Input: dimensioned drawing with shaded views. Units: mm. Origin: part minimum x, y, z. Give positions to 0.01 mm unless a question says otherwise; leave off trailing zeros. Write each loop counter-clockwise with the first axis right and the second up, starting at its lowest first coordinate (ties: lowest second). Pieces come first, ordered by that corner, then holes. Notation, with made-up numbers: (7.5, 6) -> (23.5, 6) arc R28 cw to (23.5, 29) -> close; hole circle Ø4 at (75, -8). An arc over 180 degrees is marked (long way). Answer as a JSON object with one key per item and string values.
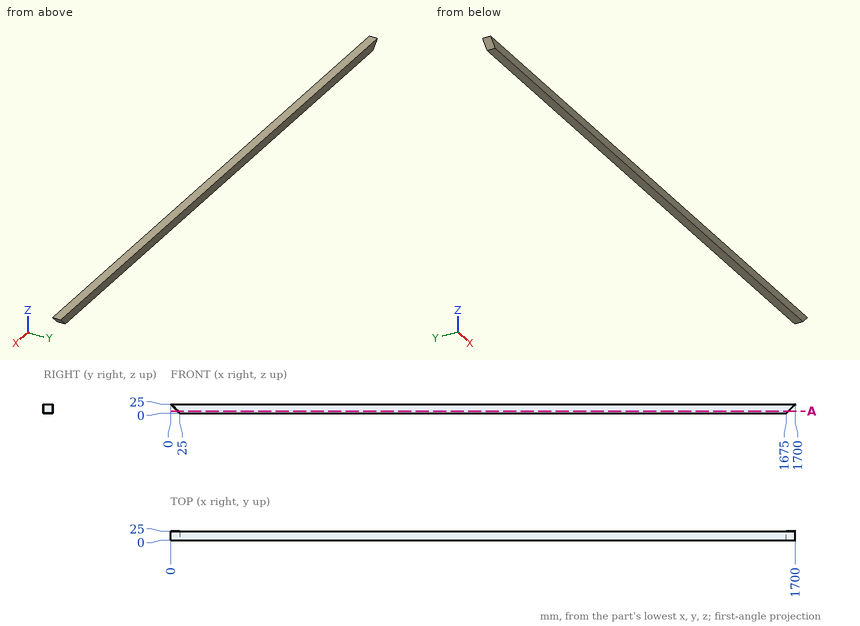
Q1. Material intervals for L1, parallel to X at y = 17, z = 23.25; L2, parallel to X at y = 5.5, z = 8.5, sorted ascending. Write a range as from..to.
Values:
{"L1": "1.75..1698.25", "L2": "16.5..1683.5"}
Q2. First-contact query: P1, Ø12, axis at y = 20.5, z = 18.5, coming from the -X side; P2, Ø2, axis at y = 14, z = 18.5, coming from the -X side; P3, Ø8, axis at y = 10.5, z = 7.5, coming from the -X side. Flat tips, straight axial feed; report the tip coordinate or a pass-through.
Values:
{"P1": "x = 0.5", "P2": "x = 5.5", "P3": "x = 13.5"}
Q3. Cut plane A-A (z = 5.75). Return the cut outline in (x, y), and give its area (3 significant figures).
Values:
{"outline": "(19.25, 0) -> (1680.75, 0) -> (1680.75, 25) -> (19.25, 25) -> close", "area": "41,500 mm²"}
